from build123d import *

# Parameters (mm, degrees)
F3_D         = 8.4328
F3_DEPTH     = 45
F3_TIP       = 2.5334687141
F2_R         = 25
F4_DEPTH     = 15
F5_T4_DEPTH  = 11.8738635424
F5_S5_R      = 8.25
F5_T6_DEPTH  = 8
F5_T10_DEPTH = 11.8738635424
F5_S11_R     = 8.25
F5_T12_DEPTH = 7
F5_T16_DEPTH = 11.8738635424
F5_S17_R     = 8.25
F5_T18_DEPTH = 8
F5_T22_DEPTH = 11.8738635424
F5_S23_R     = 8.25
F5_T24_DEPTH = 7
F5_T28_DEPTH = 11.8738635424
F5_S29_R     = 8.25
F5_T30_DEPTH = 8
F5_T34_DEPTH = 11.8738635424
F5_S35_R     = 8.25
F5_T36_DEPTH = 8
F6_SIZE      = 1
F7_R         = 3


# Not quite as in the source:
# - a fillet or chamfer that OpenCascade refuses, or shapes differently, is made with other operations: its cross-section is extruded or revolved along the edge and cut away or added


with BuildPart() as f1:
    # F0 (on Front) → F1 (revolve)
    with BuildSketch(Plane.XZ):
        Polygon((30, 8.25), (30, 0), (130, 0), (130, 4.7625), (85, 4.7625), (85, 8.25), align=None)
    revolve(axis=Axis((80, 0, 0), (-1, 0, 0)))

    # F3
    with Locations(Plane(origin=(30, 0, 0), x_dir=(0, -1, 0), z_dir=(-1, 0, 0))):
        with Locations((0, 0)):
            Hole(F3_D / 2, depth=F3_DEPTH)
            with Locations((0, 0, -(F3_DEPTH + F3_TIP / 2))):  # 118° drill point
                Cone(0, F3_D / 2, F3_TIP, mode=Mode.SUBTRACT)

    # F2 (on face) → F4 (cut)
    with BuildSketch(Plane(origin=(30, 0, 0), x_dir=(0, -1, 0), z_dir=(-1, 0, 0))):
        Circle(F2_R)
        with BuildLine():
            Line((6.7264702249, 4.7767246428), (7.5, 4.3301270189))
            Line((7.5, 4.3301270189), (7.5, 3.4369317712))
            ThreePointArc((7.5, 3.4369317712), (8.0603194726, 1.7589059099), (8.25, 0))
            ThreePointArc((8.25, 0), (8.0603194726, -1.7589059099), (7.5, -3.4369317712))
            Line((7.5, -3.4369317712), (7.5, -4.3301270189))
            Line((7.5, -4.3301270189), (6.7264702249, -4.7767246428))
            ThreePointArc((6.7264702249, -4.7767246428), (4.125, -7.1447095812), (0.7735297751, -8.213656414))
            Line((0.7735297751, -8.213656414), (0, -8.6602540378))
            Line((0, -8.6602540378), (-0.7735297751, -8.213656414))
            ThreePointArc((-0.7735297751, -8.213656414), (-4.125, -7.1447095812), (-6.7264702249, -4.7767246428))
            Line((-6.7264702249, -4.7767246428), (-7.5, -4.3301270189))
            Line((-7.5, -4.3301270189), (-7.5, -3.4369317712))
            ThreePointArc((-7.5, -3.4369317712), (-8.25, 0), (-7.5, 3.4369317712))
            Line((-7.5, 3.4369317712), (-7.5, 4.3301270189))
            Line((-7.5, 4.3301270189), (-6.7264702249, 4.7767246428))
            ThreePointArc((-6.7264702249, 4.7767246428), (-4.125, 7.1447095812), (-0.7735297751, 8.213656414))
            Line((-0.7735297751, 8.213656414), (0, 8.6602540378))
            Line((0, 8.6602540378), (0.7735297751, 8.213656414))
            ThreePointArc((0.7735297751, 8.213656414), (4.125, 7.1447095812), (6.7264702249, 4.7767246428))
        make_face(mode=Mode.SUBTRACT)
        with BuildLine():
            ThreePointArc((8.25, 0), (8.0603194726, 1.7589059099), (7.5, 3.4369317712))
            Line((7.5, 3.4369317712), (7.5, -3.4369317712))
            ThreePointArc((7.5, -3.4369317712), (8.0603194726, -1.7589059099), (8.25, 0))
        make_face()
        with BuildLine():
            Line((0.7735297751, 8.213656414), (6.7264702249, 4.7767246428))
            ThreePointArc((6.7264702249, 4.7767246428), (4.125, 7.1447095812), (0.7735297751, 8.213656414))
        make_face()
        with BuildLine():
            ThreePointArc((0.7735297751, -8.213656414), (4.125, -7.1447095812), (6.7264702249, -4.7767246428))
            Line((6.7264702249, -4.7767246428), (0.7735297751, -8.213656414))
        make_face()
        with BuildLine():
            Line((-6.7264702249, 4.7767246428), (-0.7735297751, 8.213656414))
            ThreePointArc((-0.7735297751, 8.213656414), (-4.125, 7.1447095812), (-6.7264702249, 4.7767246428))
        make_face()
        with BuildLine():
            ThreePointArc((-6.7264702249, -4.7767246428), (-4.125, -7.1447095812), (-0.7735297751, -8.213656414))
            Line((-0.7735297751, -8.213656414), (-6.7264702249, -4.7767246428))
        make_face()
        with BuildLine():
            Line((-7.5, -3.4369317712), (-7.5, 3.4369317712))
            ThreePointArc((-7.5, 3.4369317712), (-8.25, 0), (-7.5, -3.4369317712))
        make_face()
    extrude(amount=-F4_DEPTH, mode=Mode.SUBTRACT)

    # F5: fillet of radius 1 on 6 edges, made by hand


with BuildPart() as f5_tool2:
    # F5_s3 → F5_t4 (new body)
    with BuildSketch(Plane(origin=(0, 5.1415337344, 2.9684658856), x_dir=(1, 0, 0), z_dir=(0, -0.8660254038, -0.5))):
        with BuildLine():
            ThreePointArc((44, 7.5), (44.7071067812, 7.7928932188), (45, 8.5))
            Line((45, 8.5), (45, 7.5))
            Line((45, 7.5), (44, 7.5))
        make_face()
    extrude(amount=F5_T4_DEPTH)

    # F5_s5 → F5_t6 (intersect, symmetric)
    with BuildSketch(Plane.YZ.offset(44.5)):
        Circle(F5_S5_R)
    extrude(amount=F5_T6_DEPTH, both=True, mode=Mode.INTERSECT)


with BuildPart() as f1_1:
    add(f1.part)

    # F5_t1: union F5_tool2
    add(f5_tool2.part)


with BuildPart() as f5_tool8:
    # F5_s9 → F5_t10 (new body)
    with BuildSketch(Plane.XY.offset(5.9369317712)):
        with BuildLine():
            ThreePointArc((44, -7.5), (44.7071067812, -7.7928932188), (45, -8.5))
            Line((45, -8.5), (45, -7.5))
            Line((45, -7.5), (44, -7.5))
        make_face()
    extrude(amount=-F5_T10_DEPTH)

    # F5_s11 → F5_t12 (intersect, symmetric)
    with BuildSketch(Plane.YZ.offset(44.5)):
        Circle(F5_S11_R)
    extrude(amount=F5_T12_DEPTH, both=True, mode=Mode.INTERSECT)


with BuildPart() as f1_2:
    add(f1_1.part)

    # F5_t7: union F5_tool8
    add(f5_tool8.part)


with BuildPart() as f5_tool14:
    # F5_s15 → F5_t16 (new body)
    with BuildSketch(Plane(origin=(0, 5.1415337344, -2.9684658856), x_dir=(1, 0, 0), z_dir=(0, -0.8660254038, 0.5))):
        with BuildLine():
            ThreePointArc((44, 7.5), (44.7071067812, 7.7928932188), (45, 8.5))
            Line((45, 8.5), (45, 7.5))
            Line((45, 7.5), (44, 7.5))
        make_face()
    extrude(amount=F5_T16_DEPTH)

    # F5_s17 → F5_t18 (intersect, symmetric)
    with BuildSketch(Plane.YZ.offset(44.5)):
        Circle(F5_S17_R)
    extrude(amount=F5_T18_DEPTH, both=True, mode=Mode.INTERSECT)


with BuildPart() as f1_3:
    add(f1_2.part)

    # F5_t13: union F5_tool14
    add(f5_tool14.part)


with BuildPart() as f5_tool20:
    # F5_s21 → F5_t22 (new body)
    with BuildSketch(Plane.XY.offset(-5.9369317712)):
        with BuildLine():
            ThreePointArc((44, 7.5), (44.7071067812, 7.7928932188), (45, 8.5))
            Line((45, 8.5), (45, 7.5))
            Line((45, 7.5), (44, 7.5))
        make_face()
    extrude(amount=F5_T22_DEPTH)

    # F5_s23 → F5_t24 (intersect, symmetric)
    with BuildSketch(Plane.YZ.offset(44.5)):
        Circle(F5_S23_R)
    extrude(amount=F5_T24_DEPTH, both=True, mode=Mode.INTERSECT)


with BuildPart() as f1_4:
    add(f1_3.part)

    # F5_t19: union F5_tool20
    add(f5_tool20.part)


with BuildPart() as f5_tool26:
    # F5_s27 → F5_t28 (new body)
    with BuildSketch(Plane(origin=(0, -5.1415337344, -2.9684658856), x_dir=(1, 0, 0), z_dir=(0, 0.8660254038, 0.5))):
        with BuildLine():
            ThreePointArc((44, 7.5), (44.7071067812, 7.7928932188), (45, 8.5))
            Line((45, 8.5), (45, 7.5))
            Line((45, 7.5), (44, 7.5))
        make_face()
    extrude(amount=F5_T28_DEPTH)

    # F5_s29 → F5_t30 (intersect, symmetric)
    with BuildSketch(Plane.YZ.offset(44.5)):
        Circle(F5_S29_R)
    extrude(amount=F5_T30_DEPTH, both=True, mode=Mode.INTERSECT)


with BuildPart() as f1_5:
    add(f1_4.part)

    # F5_t25: union F5_tool26
    add(f5_tool26.part)


with BuildPart() as f5_tool32:
    # F5_s33 → F5_t34 (new body)
    with BuildSketch(Plane(origin=(0, -5.1415337344, 2.9684658856), x_dir=(1, 0, 0), z_dir=(0, 0.8660254038, -0.5))):
        with BuildLine():
            ThreePointArc((44, 7.5), (44.7071067812, 7.7928932188), (45, 8.5))
            Line((45, 8.5), (45, 7.5))
            Line((45, 7.5), (44, 7.5))
        make_face()
    extrude(amount=F5_T34_DEPTH)

    # F5_s35 → F5_t36 (intersect, symmetric)
    with BuildSketch(Plane.YZ.offset(44.5)):
        Circle(F5_S35_R)
    extrude(amount=F5_T36_DEPTH, both=True, mode=Mode.INTERSECT)


with BuildPart() as f1_6:
    add(f1_5.part)

    # F5_t31: union F5_tool32
    add(f5_tool32.part)

    # F6
    f6_edges = [f1_6.edges().sort_by_distance(p)[0] for p in [
        (130, 0, -4.7625),
    ]]
    chamfer(f6_edges, length=F6_SIZE)

    # F7
    f7_edges = [f1_6.edges().sort_by_distance(p)[0] for p in [
        (85, 0, -4.7625),
    ]]
    fillet(f7_edges, radius=F7_R)


solid = f1_6.part
The listing builds one solid part. Answer for the finished solid, in the listing's coordinates (mm). A direction names the side the tool comes from. Round coordinates to 2 decimals unless told otherwise and drop trailing zeros. Write each loop counter-clockwise with the first axis right and the second up, starting at its lowest first coordinate (ties: lowest second). Pieces come first, ordered by that corner, then holes. Notation, with made-up numbers: (-24, -29) - (6, -29) arc R34 ccw to (6, 4) - close; hole circle Ø4 at (6, 6). An arc over 180 degrees is marked (long way). Use one line per item in the form item = value. Start each with the question number.
Item 1: A tool of negligible diameter and unlimited length cuts with its end or side. For faces 5 (the flat face through (37, -7.5, 0)), 6 (the flat face through (36.9, 3.71, -6.52)), 7 (the flat face through (37, 7.5, 0)), 8 (the flat face through (36.9, -3.79, -6.47)), 9 (the flat face through (36.9, 3.79, 6.47)), from which of +Z, -Z, +X, -X, +Y, -Y can it reach the whole face along a straight path? Write none if from no direction.
Item 2: Flat-ended cylindrical pins translate along their axes: pin 1 Ø8 at (x, y) = (105, -4) entering from +Z; pin 2 Ø5.5 at (x, z) = (39.5, 0) entering from -Y; pin 3 Ø1 at (x, z) = (68, -1.5) entering from +Y. Find the tip coordinate at first contact, or state that the pin passes through.
Item 3: Find the intervals of material crossed by line 1 (Y direction, x = 55.5, z = 0); line 2 (Y direction, x = 63, z = 4.75), in increasing order. Write a range as [from, to].
Item 4: Determine the mould class of faces 1 (the cylindrical face through (108.21, -2.9, -3.78)), 2 (the cylindrical face through (52.82, -0.55, 4.18)), 3 (the flat face through (36.9, -3.71, 6.52)), 4 (the conical face through (77.093, 0.159, -0.715)) for opening direction Z: +Z half, -Z half, draft (parallel to the pull), parting line (faces both ways), or undercut.
Item 5: A cutting plane is placed at A-A (x = 46). Write down the section's boundary in (y, z).
Item 6: A cutting plane is placed at B-B (x = 111). Write down the section's boundary in (y, z) (1 decimal).
The answers:
q1.face_5 = +Z, -Z, -X, -Y
q1.face_6 = -Z, -X, +Y
q1.face_7 = +Z, -Z, -X, +Y
q1.face_8 = -Z, -X, -Y
q1.face_9 = +Z, -X, +Y
q2.pin_1 = 4.76
q2.pin_2 = -7.5
q2.pin_3 = 8.19
q3.line_1 = [-8.25, -4.22], [4.22, 8.25]
q3.line_2 = [-6.75, 6.75]
q4.face_1 = parting line
q4.face_2 = undercut
q4.face_3 = +Z half
q4.face_4 = undercut
q5.outline = circle Ø16.5 at (0, 0); hole circle Ø8.43 at (0, 0)
q6.outline = circle Ø9.5 at (0, 0)
